Can you work these out from the model? Positions are in its coordinate system, mm. A direction names the side the tool comes from. Give positions to 0.01 mm unless a question says otherwise; leave off trailing zeros. Order: outer loops, then holes, each group sorted by start corner. A loop starts at its lowest first (then second) coordinate and runs counter-clockwise, first axis right, second up. Notation, with made-up numbers: (-35, 10) -> (-19, 10) arc R26 ccw to (-19, 37) -> close; hole circle Ø3 at (-37, -13). An arc over 180 degrees is marked (long way). Answer as CSV lines item,"result".
Autodesk Inventor part; units mm, degrees
ref_plane "YZ Plane" through (0, 0, 0) normal (1, 0, 0) x (0, 1, 0)
ref_plane "XZ Plane" through (0, 0, 0) normal (0, 1, 0) x (-1, 0, 0)
ref_plane "XY Plane" through (0, 0, 0) normal (0, 0, 1) x (1, 0, 0)
sketch "Sketch1" plane through (0, 0, 0) normal (0, 1, 0) x (-1, 0, 0)
  line L0 (0, 0) -> (-88.9, 0)
  line L1 (-88.9, 0) -> (-88.9, -52.1)
  line L2 (-88.9, -52.1) -> (0, -52.1)
  line L3 (0, -52.1) -> (0, 0)
  dimension "d0" = 88.9
  dimension "d1" = 52.1
extrude "Extrusion1" add sketch "Sketch1" along normal blind 2.5
sketch "Sketch2" plane through (0, 2.5, 0) normal (0, 1, 0) x (1, 0, 0)
  circle A0 centre (7.6, 26.05) radius 4
  circle A1 centre (81.3, 26.05) radius 4
  line L0 (0, 52.1) -> (0, 0)
  line L1 (88.9, 0) -> (88.9, 52.1)
  line L2 (88.9, 52.1) -> (0, 52.1)
  dimension "d4" = 8
  dimension "d5" = 8
  dimension "d6" = 7.6
  dimension "d7" = 7.6
  dimension "d8" = 26.05
  dimension "d9" = 26.05
extrude "Extrusion2" add sketch "Sketch2" along normal blind 4
sketch "Sketch3" plane through (7.6, 6.5, -26.05) normal (0, 1, 0) x (1, 0, 0)
  circle A0 centre (0, 0) radius 4
  circle A1 centre (73.7, 0) radius 4
  circle A2 centre (0, 0) radius 2.25
  circle A3 centre (73.7, 0) radius 2.25
  point P0 (-7.6, -26.05)
  dimension "d12" = 4.5
  dimension "d13" = 4.5
extrude "Extrusion3" cut sketch "Sketch3" against normal blind 4.2 contours A2 | A3
chamfer "Chamfer1" distance 1.5 angle 45 2 edges at (77.3, 2.5, -26.05) (3.6, 2.5, -26.05)
fillet "Fillet1" radius 2 4 edges at (0, 1.25, 0) (88.9, 1.25, 0) (88.9, 1.25, -52.1) (0, 1.25, -52.1)
properties part number "medium_backplate"
Item 1: Imagine slicing it at A-A, the plane y = 5.5. Please give me the cut outline in (x, z).
Numbers:
outline,"circle Ø8 at (7.6, -26.05); circle Ø8 at (81.3, -26.05); hole circle Ø4.5 at (7.6, -26.05); hole circle Ø4.5 at (81.3, -26.05)"
Item 2: We'd pull the mould along Z, two halves only. Please class faces 1 (the flat face through (9, 6.5, -24)), 2 (the flat face through (44, 1, 0)), 3 (the flat face through (8, 2.3, -26)): released by +Z, released by -Z, zero draft, split by the parting line, or undercut.
Numbers:
face 1,"zero draft"
face 2,"released by +Z"
face 3,"undercut"
Item 3: Imagine slicing it at C-C, the plane x = 7.6. Please give me the cut outline in (y, z).
Numbers:
outline,"(0, -52.1) -> (2.5, -52.1) -> (2.5, -31.55) -> (4, -30.05) -> (6.5, -30.05) -> (6.5, -28.3) -> (2.3, -28.3) -> (2.3, -23.8) -> (6.5, -23.8) -> (6.5, -22.05) -> (4, -22.05) -> (2.5, -20.55) -> (2.5, 0) -> (0, 0) -> close"
Item 4: Imagine slicing it at D-D, the plane z = -47.5. Please give me the cut outline in (x, y), then the cut area to 3 significant figures.
Numbers:
outline,"(0, 0) -> (88.9, 0) -> (88.9, 2.5) -> (0, 2.5) -> close"
area,"222 mm²"
Item 5: For pin 1 (3 mm diameter, centred on x = 47.5, z = -40.5, fed in from +Y); pin 2 (4 mm diameter, centred on x = 81.3, z = -26.05, fed in from +Y), each with a flat end and sliding along its axis, tell me the tip position at first contact or that it passes through.
Numbers:
pin 1,"stops at y = 2.5"
pin 2,"stops at y = 2.3"
Item 6: For faces 4 (the flat face through (88.9, 1, -26)), 5 (the cylindrical face through (9.75, 5.232, -22.677)), which set-ups out of +Z, -Z, +X, -X, +Y, -Y let a thin tool reach every point of the face, with its end or its side?
Numbers:
face 4,"+Z, -Z, +X, +Y, -Y"
face 5,"+Y"
Item 7: Please list where these lines run through material, in increasing order: line 1 along X through (y, z) = (5.4, -26.05); line 2 along X through (y, z) = (3.8, -26.05); line 3 along Z through (x, y) = (81.3, 4.95).
Numbers:
line 1,"x = 3.6 to 5.35, 9.85 to 11.6, 77.3 to 79.05, 83.55 to 85.3"
line 2,"x = 3.4 to 5.35, 9.85 to 11.8, 77.1 to 79.05, 83.55 to 85.5"
line 3,"z = -30.05 to -28.3, -23.8 to -22.05"
Item 8: Imagine slicing it at B-B, the plane z = -26.05. Please give me the cut outline in (x, y).
Numbers:
outline,"(0, 0) -> (88.9, 0) -> (88.9, 2.5) -> (86.8, 2.5) -> (85.3, 4) -> (85.3, 6.5) -> (83.55, 6.5) -> (83.55, 2.3) -> (79.05, 2.3) -> (79.05, 6.5) -> (77.3, 6.5) -> (77.3, 4) -> (75.8, 2.5) -> (13.1, 2.5) -> (11.6, 4) -> (11.6, 6.5) -> (9.85, 6.5) -> (9.85, 2.3) -> (5.35, 2.3) -> (5.35, 6.5) -> (3.6, 6.5) -> (3.6, 4) -> (2.1, 2.5) -> (0, 2.5) -> close"
